from build123d import *

# Parameters (mm, degrees)
BOSS_EXTRUDE1_DEPTH      = 304.8
M5_CLEARANCE_HOLE1_D     = 5.5
M5_CLEARANCE_HOLE1_DEPTH = 25.4
M5_CLEARANCE_HOLE1_TIP   = 1.652366702


with BuildPart() as part:
    # Sketch1 → Boss-Extrude1 (new body)
    with BuildSketch(Plane.XY):
        Polygon((0, 0), (0, 31.75), (3.175, 31.75), (3.175, 3.175), (31.75, 3.175), (31.75, 0), align=None)
    extrude(amount=BOSS_EXTRUDE1_DEPTH)

    # M5 Clearance Hole1
    with Locations(Plane(origin=(0, 3.175, 0), x_dir=(1, 0, 0), z_dir=(0, 1, 0))):
        with Locations((19.05, -10), (19.05, -294.8), (19.05, -30), (19.05, -274.8)):
            Hole(M5_CLEARANCE_HOLE1_D / 2, depth=M5_CLEARANCE_HOLE1_DEPTH)
            with Locations((0, 0, -(M5_CLEARANCE_HOLE1_DEPTH + M5_CLEARANCE_HOLE1_TIP / 2))):  # 118° drill point
                Cone(0, M5_CLEARANCE_HOLE1_D / 2, M5_CLEARANCE_HOLE1_TIP, mode=Mode.SUBTRACT)


solid = part.part
Read the model definition and answer for the solid it produces. Units are mm, in the model's axes. A direction names the side the tool comes from. Coordinates: 2 decimals unless noted, no trailing zeros. Loops run counter-clockwise (first coordinate to the right, second up) from the corner with the lowest first, then second, coordinate; pieces in that order, holes last. Notation, with made-up numbers: (83.25, 16) -> (97.25, 16) arc R19 ccw to (97.25, 26) -> close; hole circle Ø2 at (-32.75, 70.5). An arc over 180 degrees is marked (long way). Write item = value, one per line. Start each with the question number.
1) The part is cut by section B-B, the plane z = 30. Determine the outline of the cut face in (x, y) (3 decimals), plus the area to 3 significant figures.
2) Find the intervals of material crossed by L1, parallel to Z at x = 19.05, y = 1.7; L2, parallel to X at y = 1, z = 30; L3, parallel to Y at x = 19.5, z = 14 (3 decimals), in increasing order. Write a range as from..to.
3) For faces 4 (the face through (16, 0, 150)), 5 (the face through (3.175, 18, 150)), determine the directions among +Z, -Z, +X, -X, +Y, -Y from which every point of the face is accessible in a straight line to the end or side of a thin tool.
4) The part is cut by section A-A, the plane x = 19.05. Determine the outline of the cut face in (y, z) (3 decimals), plus the area to 3 significant figures.
5) Given P1, Ø4, axis at y = 23.5, z = 120, coming from the +X side (3 decimals); P2, Ø14.5, axis at x = 24.5, z = 211, coming from the +Y side (3 decimals), each flat-ended and moving along its own axis, determine where each tip first touches the part or whether it passes through.
6) The mould has two halves that part along X. Classify faces 1 (the face through (9, 3, 0)), 2 (the face through (0, 16, 150)), 3 (the face through (16.51, 1.57, 11.05)): pulls with the +X half, pulls with the -X half, needs draft (parallel to the pull), parting line crosses it, or undercut.
7) The part is cut by section C-C, the plane y = 8.5. Determine the outline of the cut face in (x, z) (3 decimals).
Result:
q1.outline = (0, 0) -> (16.3, 0) -> (16.3, 3.175) -> (3.175, 3.175) -> (3.175, 31.75) -> (0, 31.75) -> close; (21.8, 0) -> (31.75, 0) -> (31.75, 3.175) -> (21.8, 3.175) -> close
q1.area = 174 mm²
q2.L1 = 0..7.25, 12.75..27.25, 32.75..272.05, 277.55..292.05, 297.55..304.8
q2.L2 = 0..16.3, 21.8..31.75
q2.L3 = 0..3.175
q3.face_4 = +Z, -Z, +X, -X, -Y
q3.face_5 = +Z, -Z, +X, +Y
q4.outline = (0, 0) -> (3.175, 0) -> (3.175, 7.25) -> (0, 7.25) -> close; (0, 12.75) -> (3.175, 12.75) -> (3.175, 27.25) -> (0, 27.25) -> close; (0, 32.75) -> (3.175, 32.75) -> (3.175, 272.05) -> (0, 272.05) -> close; (0, 277.55) -> (3.175, 277.55) -> (3.175, 292.05) -> (0, 292.05) -> close; (0, 297.55) -> (3.175, 297.55) -> (3.175, 304.8) -> (0, 304.8) -> close
q4.area = 898 mm²
q5.P1 = 3.175
q5.P2 = 3.175
q6.face_1 = needs draft
q6.face_2 = pulls with the -X half
q6.face_3 = undercut
q7.outline = (0, 0) -> (3.175, 0) -> (3.175, 304.8) -> (0, 304.8) -> close
